```python
from build123d import *

# Parameters (mm, degrees)
FILLET1_R = 3.175


with BuildPart() as part:
    # Sketch1 → Revolve1 (revolve)
    with BuildSketch(Plane.XY):
        Polygon((15.875, 0), (15.875, 1.031875), (18.7325, 1.031875), (15.875, 3.889375), (15.875, 4.92125), (18.7325, 4.92125), (15.875, 7.77875), (15.875, 8.810625), (18.7325, 8.810625), (15.875, 11.668125), (15.875, 12.7), (20.6375, 12.7), (20.6375, 17.4625), (0, 17.4625), (0, 12.7), (14.9225, 12.7), (14.9225, 0), align=None)
    revolve(axis=Axis((0, 0, 0), (0, 1, 0)))

    # Fillet1
    fillet1_edges = [part.edges().sort_by_distance(p)[0] for p in [
        (-20.6375, 17.4625, 0),
    ]]
    fillet(fillet1_edges, radius=FILLET1_R)


solid = part.part
```
The model under review builds one solid part; all positions refer to its coordinate system, in mm. A direction names the side the tool comes from. Coordinates: 2 decimals unless noted, no trailing zeros. Order: outer loops, then holes, each group sorted by start corner. A loop starts at its lowest first (then second) coordinate and runs counter-clockwise, first axis right, second up. Notation, with made-up numbers: (-36.5, -21) -> (-23.5, -21) arc R34 cw to (-23.5, 9) -> close; hole circle Ø6 at (16, 40.25). An arc over 180 degrees is marked (long way). Answer in a Markdown table with one row per item. Add a question column.
Item 1: Machinability: for faces 1 (the flat face through (0, 12.7, 0)), 2 (the flat face through (0, 17.462, 0)), 3 (the cylindrical face through (-3.441, 4.413, 15.497)), which of the approach directions +Z, -Z, +X, -X, +Y, -Y give a long, thin tool a straight path to every point of the face, cutting with its end or side? Answer none if there is none.
Item 2: We need section C-C on y = 7. Write out the cut boundary in (x, z) (1 decimal), plus the area to 3 significant figures.
Item 3: Clearance check with flat-ended pins moving along their axes: pin 1 (5 mm diameter, centred on x = -2.5, z = -6, fed in from -Y); pin 2 (1.5 mm diameter, centred on y = 15.5, z = -7.5, fed in from +X); pin 3 (15 mm diameter, centred on x = 4, z = -7, fed in from -Y); pin 4 (2 mm diameter, centred on x = 15, y = 7.5, fed in from -Z). State where each tip first meets the part, or that it passes through.
Item 4: We need section D-D on y = 3.25. Write out the cut boundary in (x, z) (1 decimal), plus the area to 3 significant figures.
Item 5: To check wall thickness, follow probe 1 along Y at (x, z) = (-13, -10.5); probe 2 along Y at (x, z) = (11, -10); probe 3 along Y at (x, z) = (-12.5, -13.5). State the ranges of each line that lie inside material, in increasing order.
Item 6: Mouldability with a two-part tool opening along Y and no side actions: class faces 4 (the conical face through (-3.47, 11.53, 15.63)), 5 (the flat face through (14, 1.032, -8)), 6 (the flat face through (14, 4.921, -8)), 7 (the cylindrical face through (14.233, 6.261, -4.482)) as +Y half, -Y half, draft (parallel to the pull), parting line (faces both ways), or undercut.
Final values:
| question | item | result |
|---|---|---|
| 1 | face 1 | -Y |
| 1 | face 2 | +Z, -Z, +X, -X, +Y |
| 1 | face 3 | none |
| 2 | outline | circle Ø33.3 at (0, 0); hole circle Ø29.8 at (0, 0) |
| 2 | area | 172 mm2 |
| 3 | pin 1 | stops at y = 12.7 |
| 3 | pin 2 | stops at x = 19.35 |
| 3 | pin 3 | stops at y = 0 |
| 3 | pin 4 | stops at z = -8.95 |
| 4 | outline | circle Ø33 at (0, 0); hole circle Ø29.8 at (0, 0) |
| 4 | area | 157 mm2 |
| 5 | probe 1 | y = 1.03 to 3.05, 4.92 to 6.94, 8.81 to 10.83, 12.7 to 17.46 |
| 5 | probe 2 | y = 12.7 to 17.46 |
| 5 | probe 3 | y = 1.03 to 1.37, 4.92 to 5.26, 8.81 to 9.14, 12.7 to 17.32 |
| 6 | face 4 | undercut |
| 6 | face 5 | -Y half |
| 6 | face 6 | undercut |
| 6 | face 7 | draft |
